from build123d import *

# Parameters (mm, degrees)
SKETCH1_R           = 15.494
BOSS_EXTRUDE1_DEPTH = 25.4
BOSS_EXTRUDE2_START = -7.4168
BOSS_EXTRUDE2_DEPTH = 7.4168
BOSS_EXTRUDE4_DEPTH = 25.4
CUT_EXTRUDE1_DEPTH  = 92.576032231


with BuildPart() as part:
    # Sketch1 → Boss-Extrude1 (new body)
    with BuildSketch(Plane.XY):
        Circle(SKETCH1_R)
    extrude(amount=-BOSS_EXTRUDE1_DEPTH)

    # Sketch2 → Boss-Extrude2 (add)
    with BuildSketch(Plane(origin=(0, 0, -25.4), x_dir=(-1, 0, 0), z_dir=(0, 0, -1)).offset(BOSS_EXTRUDE2_START)):
        with BuildLine():
            Line((-15.494, 0), (-15.494, 25.4))
            Line((-15.494, 25.4), (15.494, 25.4))
            Line((15.494, 25.4), (15.494, 0))
            ThreePointArc((15.494, 0), (0, 15.494), (-15.494, 0))
        make_face()
    extrude(amount=BOSS_EXTRUDE2_DEPTH)

    # Sketch3 → Boss-Extrude4 (add)
    with BuildSketch(Plane(origin=(0, 0, -25.4), x_dir=(-1, 0, 0), z_dir=(0, 0, -1))):
        Polygon((-15.494, 25.4), (-40.894, 25.4), (-40.894, 77.9018), (40.894, 77.9018), (40.894, 25.4), (15.494, 25.4), align=None)
    extrude(amount=-BOSS_EXTRUDE4_DEPTH)

    # Sketch4 → Cut-Extrude1 (cut, through all)
    with BuildSketch(Plane(origin=(0, 0, -25.4), x_dir=(-1, 0, 0), z_dir=(0, 0, -1))):
        Polygon((-5.94478872, 77.9018), (-5.94478872, 54.1274), (-17.8308, 54.1274), (-17.8308, 37.2872), (17.8308, 37.2872), (17.8308, 54.1274), (5.9554872, 54.1274), (5.9554872, 77.9018), align=None)
    extrude(amount=-CUT_EXTRUDE1_DEPTH, mode=Mode.SUBTRACT)


solid = part.part
Geometry: final body of the model. Coordinates: model frame, mm. A direction names the side the tool comes from. Coordinates: 2 decimals unless noted, no trailing zeros. Order: outer loops, then holes, each group sorted by start corner. A loop starts at its lowest first (then second) coordinate and runs counter-clockwise, first axis right, second up.
(1) Section query A-A (z = -4.25). Return the cut outline in (x, y).
(2) Section query C-C (x = 0). Return the cut outline in (y, z).
(3) Section query D-D (z = -20.25). Return the cut outline in (x, y).
(4) Section query B-B (y = 70). Return the cut outline in (x, z).
(5) Draft query along X for faces 4 (the face through (0, 37.287, -13)), 5 (the face through (1, 25.4, -13)), 6 (the face through (15.494, 13, -22)). Return one class per face: pulls with the +X half, pulls with the -X half, needs draft (parallel to the pull), parting line crosses it, or undercut.
(6) First-contact query: pin 1 (6 mm diameter, centred on y = 8, z = -23.5, fed in from -X); pin 2 (5 mm diameter, centred on x = -19, y = 23.5, fed in from +Z); pin 3 (8 mm diameter, centred on y = 12.5, z = -21, fed in from +X); pin 4 (10 mm diameter, centred on x = 0.5, y = 44.5, fed in from -Z). Flat tips, straight axial feed; report the tip coordinate or a pass-through.
(7) Material intervals for probe 1 along X at (y, z) = (38.5, -6.25); probe 2 along Y at (x, z) = (-6, -3); probe 3 along Y at (x, z) = (13, -17), sorted ascending.
(8) Access query for faces 1 (the face through (-15.494, 13, -22)), 2 (the face through (12, 54.127, -13)), 3 (the face through (5.945, 66, -13)). Directions: +Z, -Z, +X, -X, +Y, -Y. A direction counts if a zero-diameter tool reaches every point of the face in a straight line with its end or side. Return the directions, or none.
Solution:
1. outline: (-40.89, 25.4) - (40.89, 25.4) - (40.89, 77.9) - (5.94, 77.9) - (5.94, 54.13) - (17.83, 54.13) - (17.83, 37.29) - (-17.83, 37.29) - (-17.83, 54.13) - (-5.96, 54.13) - (-5.96, 77.9) - (-40.89, 77.9) - close; circle Ø30.99 at (0, 0)
2. outline: (-15.49, -25.4) - (37.29, -25.4) - (37.29, 0) - (25.4, 0) - (25.4, -17.98) - (15.49, -17.98) - (15.49, 0) - (-15.49, 0) - close
3. outline: (-40.89, 25.4) - (-15.49, 25.4) - (-15.49, 0) arc R15.49 ccw to (15.49, 0) - (15.49, 25.4) - (40.89, 25.4) - (40.89, 77.9) - (5.94, 77.9) - (5.94, 54.13) - (17.83, 54.13) - (17.83, 37.29) - (-17.83, 37.29) - (-17.83, 54.13) - (-5.96, 54.13) - (-5.96, 77.9) - (-40.89, 77.9) - close
4. outline: (-40.89, -25.4) - (-5.96, -25.4) - (-5.96, 0) - (-40.89, 0) - close; (5.94, -25.4) - (40.89, -25.4) - (40.89, 0) - (5.94, 0) - close
5. face 4: undercut
5. face 5: needs draft
5. face 6: pulls with the +X half
6. pin 1: stops at x = -15.49
6. pin 2: stops at z = 0
6. pin 3: stops at x = 15.49
6. pin 4: passes through
7. probe 1: x = -40.89 to -17.83, 17.83 to 40.89
7. probe 2: y = -14.29 to 14.29, 25.4 to 37.29, 54.13 to 77.9
7. probe 3: y = -8.43 to 8.43, 25.4 to 37.29, 54.13 to 77.9
8. face 1: +Z, -Z, -X, -Y
8. face 2: +Z, -Z
8. face 3: +Z, -Z, +Y
